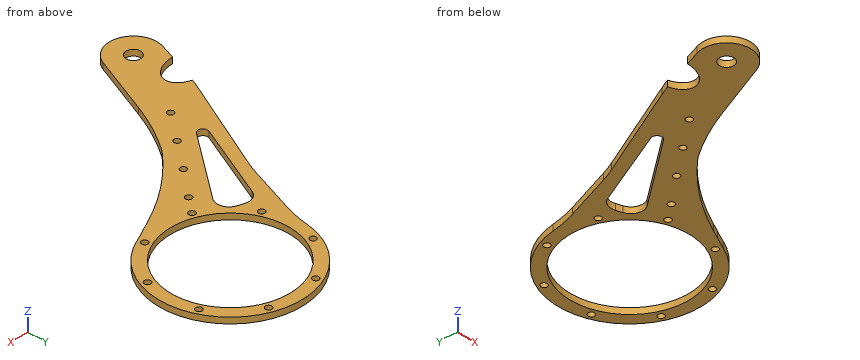
```python
from build123d import *

# Parameters (mm, degrees)
SKETCH_1_R          = 1.85
SKETCH_1_R_2        = 6
SKETCH_1_R_3        = 2.6
SKETCH_1_R_4        = 40
EXTRUDE_1_DEPTH     = 5
SKETCH_2_R          = 50
CUT_EXTRUDE_1_DEPTH = 5


with BuildPart() as part:
    # 草图1 → 凸台-拉伸1 (new body)
    with BuildSketch(Plane.XY):
        with BuildLine():
            Line((45.340426295, 11.113882118), (52.986920218, 14.612571091))
            ThreePointArc((52.986920218, 14.612571091), (57.510180634, 16.855144901), (62.140860345, 18.86656915))
            ThreePointArc((62.140860345, 18.86656915), (76.473592144, 121.843079098), (-19.812815771, 82.619152052))
            ThreePointArc((-19.812815771, 82.619152052), (-21.816180826, 72.160455141), (-24.920337213, 61.974090443))
            Line((-24.920337213, 61.974090443), (-38.992341568, 23.311576231))
            ThreePointArc((-38.992341568, 23.311576231), (-41.02904615, 18.163814554), (-43.347502102, 13.136650558))
            Line((-43.347502102, 13.136650558), (-81.294613945, -63.493156131))
            ThreePointArc((-81.294613945, -63.493156131), (-83.173683364, -67.393304084), (-84.967894718, -71.333210372))
            add(Edge.make_bspline(
                [(-94.673253721, -96.669107716), (-78.493027504, -96.908185151), (-74.407692057, -86.243392693), (-70.32235661, -75.578600234), (-84.967894718, -71.333210372)],
                knots=[1.469085418, 1.469085418, 1.469085418, 2.850930512, 2.850930512, 4.232775606, 4.232775606, 4.232775606], degree=2, weights=[1, 0.770658452, 1, 0.770658452, 1]))
            Line((-94.673253721, -96.669107716), (-99.039465007, -108.665174635))
            ThreePointArc((-99.039465007, -108.665174635), (-87.586525496, -134.109636137), (-61.84467438, -123.341741928))
            Line((-61.84467438, -123.341741928), (-41.665865642, -75.957716718))
            ThreePointArc((-41.665865642, -75.957716718), (-30.867859398, -54.330265242), (-17.539479197, -34.163513461))
            ThreePointArc((-17.539479197, -34.163513461), (11.686808966, -8.450543885), (45.340426295, 11.113882118))
        make_face()
        with Locations((84.133254342, 74.484980418)):
            Circle(SKETCH_1_R, mode=Mode.SUBTRACT)
        with Locations((-4.866745658, 74.484980418)):
            Circle(SKETCH_1_R, mode=Mode.SUBTRACT)
        with Locations((71.099506104, 43.018728655)):
            Circle(SKETCH_1_R, mode=Mode.SUBTRACT)
        with Locations((-80.245612592, -115.505577501)):
            Circle(SKETCH_1_R_2, mode=Mode.SUBTRACT)
        with Locations((71.099506104, 105.95123218)):
            Circle(SKETCH_1_R, mode=Mode.SUBTRACT)
        with Locations((39.633254342, 29.984980418)):
            Circle(SKETCH_1_R, mode=Mode.SUBTRACT)
        with Locations((8.167002579, 43.018728655)):
            Circle(SKETCH_1_R, mode=Mode.SUBTRACT)
        with Locations((8.167002579, 105.95123218)):
            Circle(SKETCH_1_R, mode=Mode.SUBTRACT)
        with Locations((39.633254342, 118.984980418)):
            Circle(SKETCH_1_R, mode=Mode.SUBTRACT)
        with Locations((90.44662863, 95.532569198)):
            Circle(SKETCH_1_R_3, mode=Mode.SUBTRACT)
        with Locations((60.680843122, 125.298354706)):
            Circle(SKETCH_1_R_3, mode=Mode.SUBTRACT)
        with Locations((18.585665562, 125.298354706)):
            Circle(SKETCH_1_R_3, mode=Mode.SUBTRACT)
        with Locations((-11.180119947, 95.532569198)):
            Circle(SKETCH_1_R_3, mode=Mode.SUBTRACT)
        with Locations((-11.180119947, 53.437391637)):
            Circle(SKETCH_1_R_3, mode=Mode.SUBTRACT)
        with Locations((18.585665562, 23.671606129)):
            Circle(SKETCH_1_R_3, mode=Mode.SUBTRACT)
        with Locations((60.680843122, 23.671606129)):
            Circle(SKETCH_1_R_3, mode=Mode.SUBTRACT)
        with Locations((90.44662863, 53.437391637)):
            Circle(SKETCH_1_R_3, mode=Mode.SUBTRACT)
        with Locations((-31.375823455, -34.648004813)):
            Circle(SKETCH_1_R_3, mode=Mode.SUBTRACT)
        with Locations((7.718202275, 10.862157861)):
            Circle(SKETCH_1_R_3, mode=Mode.SUBTRACT)
        with Locations((-12.092195165, -11.66667152)):
            Circle(SKETCH_1_R_3, mode=Mode.SUBTRACT)
        with Locations((-50.659451746, -57.629338107)):
            Circle(SKETCH_1_R_3, mode=Mode.SUBTRACT)
        with Locations((39.633254342, 74.484980418)):
            Circle(SKETCH_1_R_4, mode=Mode.SUBTRACT)
        with BuildLine():
            Line((-5.536305869, 38.415363853), (-10.514583927, 40.122913857))
            ThreePointArc((-10.514583927, 40.122913857), (-17.662135878, 39.870705025), (-22.813209689, 34.909097746))
            Line((-22.813209689, 34.909097746), (-51.994954934, -27.329380157))
            ThreePointArc((-51.994954934, -27.329380157), (-50.503277554, -32.413196821), (-45.27475721, -31.55711955))
            Line((-45.27475721, -31.55711955), (-1.034437322, 22.632199259))
            ThreePointArc((-1.034437322, 22.632199259), (0.835703515, 31.699245343), (-5.536305869, 38.415363853))
        make_face(mode=Mode.SUBTRACT)
    extrude(amount=EXTRUDE_1_DEPTH)

    # 草图2 → 切除-拉伸1 (cut)
    with BuildSketch(Plane.XY.offset(5)):
        with Locations((39.633254342, 74.484980418)):
            Circle(SKETCH_2_R)
    extrude(amount=-CUT_EXTRUDE_1_DEPTH, mode=Mode.SUBTRACT)


solid = part.part
```
Work out the finished part from the listing and answer in its coordinate system (mm). Round coordinates to 2 decimals unless told otherwise and drop trailing zeros. Loops run counter-clockwise (first coordinate to the right, second up) from the corner with the lowest first, then second, coordinate; pieces in that order, holes last.
(1) Find the intervals of material crossed by L1, parallel to X at y = 36, z = 3.5; L2, parallel to Y at x = 39.5, z = 2.85; L3, parallel to Y at x = -78, z = 3.95, in increasing order.
Computed values:
L1: x = -34.37 to -22.22, -1.68 to 7.71, 71.55 to 85.66
L2: y = 8.33 to 24.49, 124.48 to 134.48
L3: y = -135.38 to -121.07, -109.94 to -91.2, -74.86 to -56.84
(2) The part is cut by section A-A, the plane x = 83.5. Give the vertices of the cut face in (y, z), and give its area (3 significant figures).
Computed values:
outline: (33.55, 0) - (50.49, 0) - (50.49, 5) - (33.55, 5) - close; (98.48, 0) - (115.42, 0) - (115.42, 5) - (98.48, 5) - close
area: 169 mm2
(3) Each of these flat-tipped pins is pushed along its axis until it touches: P1, Ø8.5, axis at x = 60.68, y = 125.3, coming from the +Z side; P2, Ø3, axis at y = -16.5, z = 1, coming from the +X side. Where does it stop, or does it pass through?
Computed values:
P1: stops at z = 5
P2: stops at x = 3.09
(4) The part is cut by section B-B, the plane y = 48. Give the vertices of the cut face in (x, z), and give its area (3 significant figures).
Computed values:
outline: (-30.01, 0) - (-2.78, 0) - (-2.78, 5) - (-30.01, 5) - close; (82.04, 0) - (93.47, 0) - (93.47, 5) - (82.04, 5) - close
area: 193 mm2
(5) The part is cut by section C-C, the plane z = 3.8. Give the number of separate pieces and of enclosed holes in the cut face, and give its area (3 significant figures).
Computed values:
separate pieces: 1
enclosed holes: 15
area: 10,400 mm2
